from build123d import *

# Parameters (mm, degrees)
ESQUISSE1_W             = 180
ESQUISSE1_H             = 110
BOSS_EXTRU_1_DEPTH      = 5
ESQUISSE2_W             = 20
ESQUISSE2_H             = 10
ESQUISSE2_W_2           = 5
ESQUISSE2_H_2           = 25
ENL_V_MAT_EXTRU_1_DEPTH = 5


with BuildPart() as part:
    # Esquisse1 → Boss.-Extru.1 (new body)
    with BuildSketch(Plane(origin=(0, 0, 0), x_dir=(1, 0, 0), z_dir=(0, 1, 0))):
        Rectangle(ESQUISSE1_W, ESQUISSE1_H)
    extrude(amount=BOSS_EXTRU_1_DEPTH)

    # Esquisse2 → Enlèv. mat.-Extru.1 (cut)
    with BuildSketch(Plane(origin=(0, 5, 0), x_dir=(1, 0, 0), z_dir=(0, 1, 0))):
        Polygon((-90, 55), (-90, 27.5), (-85, 27.5), (-85, 45), (-50, 45), (-50, 55), align=None)
        Polygon((85, 27.5), (90, 27.5), (90, 55), (50, 55), (50, 45), (85, 45), align=None)
        with Locations((20, 50)):
            Rectangle(ESQUISSE2_W, ESQUISSE2_H)
        with Locations((-20, 50)):
            Rectangle(ESQUISSE2_W, ESQUISSE2_H)
        with Locations((-87.5, 0)):
            Rectangle(ESQUISSE2_W_2, ESQUISSE2_H_2)
        Polygon((-90, -55), (-50, -55), (-50, -45), (-85, -45), (-85, -27.5), (-90, -27.5), align=None)
        Polygon((50, -45), (50, -55), (90, -55), (90, -27.5), (85, -27.5), (85, -45), align=None)
        with Locations((87.5, 0)):
            Rectangle(ESQUISSE2_W_2, ESQUISSE2_H_2)
        with Locations((20, -50)):
            Rectangle(ESQUISSE2_W, ESQUISSE2_H)
        with Locations((-20, -50)):
            Rectangle(ESQUISSE2_W, ESQUISSE2_H)
    extrude(amount=-ENL_V_MAT_EXTRU_1_DEPTH, mode=Mode.SUBTRACT)


solid = part.part
Work out the finished part from the listing and answer in its coordinate system (mm). A direction names the side the tool comes from. Coordinates: 2 decimals unless noted, no trailing zeros. Write each loop counter-clockwise with the first axis right and the second up, starting at its lowest first coordinate (ties: lowest second). Pieces come first, ordered by that corner, then holes. Notation, with made-up numbers: M -21,52.25 L -16,52.25 A18 ccw -16,81.25 Z; hole C 72.5,9 d2. An arc over 180 degrees is marked long. Answer as CSV lines item,"result". Start each with the question number.
Item 1: Section A-A on z = 40 is taken. Write down the section's boundary in (x, y).
Item 2: Determine the mould class of faces 1 (the face through (87, 3, 12.5)), 2 (the face through (20, 3, -45)), 3 (the face through (-85, 3, 36)) for opening direction X: released by +X, released by -X, zero draft, split by the parting line, or undercut.
Item 3: A tool of negligible diameter and unlimited length cuts with its end or side. For faces 4 (the face through (50, 3, 50)), 5 (the face through (-88, 3, 12.5)), 6 (the face through (50, 3, -50)), 7 (the face through (-67, 3, 45)), 8 (the face through (30, 3, 50)), from which of +Z, -Z, +X, -X, +Y, -Y can it reach the whole face along a straight path? Write none if from no direction.
Item 4: Consider L1, parallel to X at y = 3.6, z = 50; L2, parallel to Z at x = 55, y = 1.6; L3, parallel to X at y = 1.3, z = 33.5. Determine where each line is inside the solid, lowest interval first.
Item 5: Flat-ended cylindrical pins translate along their axes: P1, Ø2.5, axis at y = 1.5, z = 52.5, coming from the -X side; P2, Ø1.5, axis at x = 70.5, y = 4, coming from the +Z side; P3, Ø1.5, axis at y = 2.5, z = 34.5, coming from the +X side. Find the tip coordinate at first contact, or state that the pin passes through.
Item 6: Section B-B on x = 74 is taken. Write down the section's boundary in (y, z), and give its area (3 significant figures).
Checks:
1,outline,"M -85,0 L 85,0 L 85,5 L -85,5 Z"
2,face 1,"zero draft"
2,face 2,"undercut"
2,face 3,"released by -X"
3,face 4,"+Z, +X, +Y, -Y"
3,face 5,"-X, +Y, -Y"
3,face 6,"-Z, +X, +Y, -Y"
3,face 7,"+Z, -X, +Y, -Y"
3,face 8,"+Z, +Y, -Y"
4,L1,"x = -50 to -30, -10 to 10, 30 to 50"
4,L2,"z = -45 to 45"
4,L3,"x = -85 to 85"
5,P1,"stops at x = -50"
5,P2,"stops at z = 45"
5,P3,"stops at x = 85"
6,outline,"M 0,-45 L 5,-45 L 5,45 L 0,45 Z"
6,area,"450 mm²"
